Build history of the part. All positions in model axes, mm. A direction names the side the tool comes from. Round coordinates to 2 decimals unless told otherwise and drop trailing zeros. Loops run counter-clockwise (first coordinate to the right, second up) from the corner with the lowest first, then second, coordinate; pieces in that order, holes last. Notation, with made-up numbers: (-24.75, 4.5) - (8.25, 4.5) arc R29 ccw to (8.25, 27.5) - close; hole circle Ø10 at (77, 77). An arc over 180 degrees is marked (long way). Put each result on its own line as item: value. Start each with the question number.
from build123d import *

# Parameters (mm, degrees)
SKETCH1_W               = 150.8
SKETCH1_H               = 131.6
BOSS_EXTRUDE1_DEPTH     = 4
F_5_0MM_DOWEL_HOLE1_D   = 5
F_5_0MM_DOWEL_HOLE2_D   = 5
CAVITY1_START           = -58.8
CAVITY1_OUTLINE_W       = 10
CAVITY1_OUTLINE_H       = 3.997862951
CAVITY1_DEPTH           = 4
CAVITY1_START_2         = -33.210330997
CAVITY1_2_OUTLINE_W     = 4
CAVITY1_2_OUTLINE_H     = 3.997862951
CAVITY1_2_DEPTH         = 10
CAVITY1_START_3         = 21.789669003
CAVITY1_3_OUTLINE_W     = 4
CAVITY1_3_OUTLINE_H     = 3.997862951
CAVITY1_3_DEPTH         = 10
CUT_EXTRUDE6_DEPTH      = 101.153796274
CUT_EXTRUDE6_DEPTH_BACK = 101.153796274
SKETCH14_W              = 4
SKETCH14_H              = 10
SKETCH14_W_2            = 10
SKETCH14_H_2            = 4
SKETCH15_W              = 10
SKETCH15_H              = 4
BOSS_EXTRUDE2_DEPTH     = 4


# Read off the part's stored shape, not the designer's step: Cavity1
with BuildPart() as part:
    # Sketch1 → Boss-Extrude1 (new body)
    with BuildSketch(Plane(origin=(0, 0, 0), x_dir=(1, 0, 0), z_dir=(0, 1, 0))):
        Rectangle(SKETCH1_W, SKETCH1_H)
    extrude(amount=BOSS_EXTRUDE1_DEPTH)

    # Ø5.0mm Dowel Hole1 (through all)
    with Locations(Plane(origin=(0, 4, 0), x_dir=(1, 0, 0), z_dir=(0, 1, 0))):
        with Locations((-42.5, -20.3)):
            Hole(F_5_0MM_DOWEL_HOLE1_D / 2)

    # Ø5.0mm Dowel Hole2 (through all)
    with Locations(Plane(origin=(0, 4, 0), x_dir=(1, 0, 0), z_dir=(0, 1, 0))):
        with Locations((-12.5, -20.3), (17.5, -20.3), (47.5, -20.3), (-47.5, 34.5), (-17.5, 34.5), (12.5, 34.5), (42.5, 34.5)):
            Hole(F_5_0MM_DOWEL_HOLE2_D / 2)

    # Cavity1 outline → Cavity1 (cut)
    with BuildSketch(Plane.XY.offset(CAVITY1_START)):
        with Locations((25.4, 2.001068524)):
            Rectangle(CAVITY1_OUTLINE_W, CAVITY1_OUTLINE_H)
        with Locations((-25.4, 2.001068524)):
            Rectangle(CAVITY1_OUTLINE_W, CAVITY1_OUTLINE_H)
    extrude(amount=CAVITY1_DEPTH, mode=Mode.SUBTRACT)

    # Cavity1 2 outline → Cavity1 2 (cut)
    with BuildSketch(Plane.XY.offset(CAVITY1_START_2)):
        with Locations((-66.4, 2.001068524)):
            Rectangle(CAVITY1_2_OUTLINE_W, CAVITY1_2_OUTLINE_H)
        with Locations((66.4, 2.001068524)):
            Rectangle(CAVITY1_2_OUTLINE_W, CAVITY1_2_OUTLINE_H)
    extrude(amount=CAVITY1_2_DEPTH, mode=Mode.SUBTRACT)

    # Cavity1 3 outline → Cavity1 3 (cut)
    with BuildSketch(Plane.XY.offset(CAVITY1_START_3)):
        with Locations((-66.4, 2.001068524)):
            Rectangle(CAVITY1_3_OUTLINE_W, CAVITY1_3_OUTLINE_H)
        with Locations((66.4, 2.001068524)):
            Rectangle(CAVITY1_3_OUTLINE_W, CAVITY1_3_OUTLINE_H)
    extrude(amount=CAVITY1_3_DEPTH, mode=Mode.SUBTRACT)

    # Sketch14 → Cut-Extrude6 (cut, two sides: drawn at the far end of the back side and taken through both)
    with BuildSketch(Plane(origin=(0, 0.002137049, 0), x_dir=(1, 0, 0), z_dir=(0, 1, 0)).offset(-CUT_EXTRUDE6_DEPTH_BACK)):
        with Locations((-66.4, -26.789669003)):
            Rectangle(SKETCH14_W, SKETCH14_H)
        with Locations((-66.4, 28.210330997)):
            Rectangle(SKETCH14_W, SKETCH14_H)
        with Locations((25.4, 56.8)):
            Rectangle(SKETCH14_W_2, SKETCH14_H_2)
        with Locations((-25.4, 56.8)):
            Rectangle(SKETCH14_W_2, SKETCH14_H_2)
        with Locations((66.4, 28.210330997)):
            Rectangle(SKETCH14_W, SKETCH14_H)
        with Locations((66.4, -26.789669003)):
            Rectangle(SKETCH14_W, SKETCH14_H)
    extrude(amount=CUT_EXTRUDE6_DEPTH + CUT_EXTRUDE6_DEPTH_BACK, mode=Mode.SUBTRACT)

    # Sketch15 → Boss-Extrude2 (add)
    with BuildSketch(Plane.XY.offset(65.8)):
        with Locations((-50, 2)):
            Rectangle(SKETCH15_W, SKETCH15_H)
        with Locations((0, 2)):
            Rectangle(SKETCH15_W, SKETCH15_H)
        with Locations((50, 2)):
            Rectangle(SKETCH15_W, SKETCH15_H)
    extrude(amount=BOSS_EXTRUDE2_DEPTH)


solid = part.part
Item 1: Drill centre lines: probe 1 along X at (y, z) = (1.75, -34.5); probe 2 along X at (y, z) = (2.6, -26); probe 3 along Z at (x, y) = (68, 1.4). Where is each one in solid material? Low to high. Write a range as [from, to].
Item 2: Slice it at A-A (x = 12.5). Give the cut face in (y, z), plus the area to 3 significant figures.
Item 3: Slice it at C-C (y = 1.95). Give the number of separate pieces and of enclosed holes in the cut face, plus the area to 3 significant figures.
Item 4: Drop flat-ended pins along their axis: pin 1 Ø2 at (y, z) = (2, 68.5) entering from +X; pin 2 Ø2 at (x, y) = (-67, 1) entering from +Z; pin 3 Ø6.5 at (x, z) = (42.5, -34.5) entering from -Y. Give the stop position or say it passes through.
Item 5: Which spindle directions (+Z, -Z, +X, -X, +Y, -Y) get a long thin tool onto all of the face, cutting with end or side? Do faces 4 (the flat face through (-65, 2, 65.8)), 5 (the flat face through (-68.4, 2, -28)), 6 (the flat face through (-1, 4, 1)), 7 (the flat face through (45, 2, 68)). Say none if no direction does.
Item 6: Two-plate mould, pull along X, no slides. Class faces 1 (the flat face through (0, 2, 69.8)), 2 (the flat face through (-30.4, 2, -57)), 3 (the cylindrical face through (19.5, 2, 21.8)): pulls with the +X half, pulls with the -X half, needs draft (parallel to the pull), parting line crosses it, or undercut.
Item 7: Slice it at B-B (x = -47.5). Give the cut face in (y, z), plus the area to 3 significant figures.
Computed values:
1. probe 1: x = [-75.4, -50], [-45, -20], [-15, 10], [15, 40], [45, 75.4]
1. probe 2: x = [-75.4, -68.4], [-64.4, 64.4], [68.4, 75.4]
1. probe 3: z = [-65.8, -33.21], [-23.21, 21.79], [31.79, 65.8]
2. outline: (0, -65.8) - (4, -65.8) - (4, -37) - (0, -37) - close; (0, -32) - (4, -32) - (4, 65.8) - (0, 65.8) - close
2. area: 506 mm^2
3. separate pieces: 1
3. enclosed holes: 14
3. area: 19,600 mm^2
4. pin 1: stops at x = 55
4. pin 2: stops at z = 65.8
4. pin 3: stops at y = 0
5. face 4: +Z, -X, +Y, -Y
5. face 5: +Y, -Y
5. face 6: +Z, -Z, +X, -X, +Y
5. face 7: +Z, +Y, -Y
6. face 1: needs draft
6. face 2: undercut
6. face 3: undercut
7. outline: (0, -65.8) - (4, -65.8) - (4, -37) - (0, -37) - close; (0, -32) - (4, -32) - (4, 69.8) - (0, 69.8) - close
7. area: 522 mm^2
